```python
from build123d import *

# Parameters (mm, degrees)
F0_R            = 63.5
F0_R_2          = 14.1605
F1_DEPTH        = 3.175
F2_R            = 2.3622
F3_DEPTH        = 3.176
F3_COPIES_COUNT = 6


# Not quite as in the source:
# - a pattern or mirror of a feature is missing from the dataset's text; its kind, count and spacing are read off the source's solid


with BuildPart() as f1:
    # F0 (on Top) → F1 (new body)
    with BuildSketch(Plane.XY):
        Circle(F0_R)
        Circle(F0_R_2, mode=Mode.SUBTRACT)
    extrude(amount=F1_DEPTH)

    # F2 (on face) → F3 (cut, through all)
    with BuildSketch(Plane.XY.offset(3.175)):
        with Locations((0, 23.8125)):
            Circle(F2_R)
        with Locations((25.4, 43.9940905122)):
            Circle(F2_R)
    f3 = extrude(amount=-F3_DEPTH, mode=Mode.SUBTRACT)

    # F3_copies: F3 ×6 about axis
    f3_copies_axis = Axis((0, 0, 0), (0, 0, 1))
    for i in range(1, F3_COPIES_COUNT):
        add(f3.rotate(f3_copies_axis, i * 360 / F3_COPIES_COUNT), mode=Mode.SUBTRACT)


solid = f1.part
```
CAD build for the part. Positions are in the model's coordinates, mm. Round coordinates to 2 decimals unless told otherwise and drop trailing zeros. Loops run counter-clockwise (first coordinate to the right, second up) from the corner with the lowest first, then second, coordinate; pieces in that order, holes last. Notation, with made-up numbers: (82, 63) - (90, 63) arc R22 cw to (90, 75) - close; hole circle Ø2 at (-32.75, 58.25). An arc over 180 degrees is marked (long way). Return JSON: item names as keys, results as strings. Group by question number.
Q1. Band-saw the part on A-A on y = 0. Give the cut face in (x, z) (1 decimal).
Q2. Band-saw the part on B-B on x = 0. Give the cut face in (y, z) (1 decimal).
Q3. Drill centre lines: line 1 along Y through (x, z) = (-25.4, 2.1); line 2 along Y through (x, z) = (20.5, 2); line 3 along X through (y, z) = (43.5, 1.3). Where is each one in solid material? Low to high. Write a range as [from, to].
Q4. Band-saw the part on D-D on y = 38. Give the cut face in (x, z) (3 decimals).
Q5. Two-plate mould, pull along X, no slides. Class faces 1 (the face through (-15, 1, 0)), 2 (the face through (-13.77, -61.99, 1.57)), 3 (the face through (0.308, -26.155, 1.61)): +X half, -X half, draft (parallel to the pull), parting line (faces both ways), or undercut.
Q6. Flat gauge pins, fed straight in: pin 1 Ø4.5 at (x, y) = (-25.4, 43.99) entering from -Z; pin 2 Ø1 at (y, z) = (41, 1) entering from -X; pin 3 Ø1.5 at (x, z) = (-12, 1) entering from +Y. Where does each tip first touch, or does it go through?
Q7. Band-saw the part on C-C on z = 0.85. Give the number of separate pieces and of enclosed holes in the cut face, plus the area to 3 significant figures.
Solutions:
{
 "1": {"outline": "(-63.5, 0) - (-53.2, 0) - (-53.2, 3.2) - (-63.5, 3.2) - close; (-48.4, 0) - (-14.2, 0) - (-14.2, 3.2) - (-48.4, 3.2) - close; (14.2, 0) - (48.4, 0) - (48.4, 3.2) - (14.2, 3.2) - close; (53.2, 0) - (63.5, 0) - (63.5, 3.2) - (53.2, 3.2) - close"},
 "2": {"outline": "(-63.5, 0) - (-26.2, 0) - (-26.2, 3.2) - (-63.5, 3.2) - close; (-21.5, 0) - (-14.2, 0) - (-14.2, 3.2) - (-21.5, 3.2) - close; (14.2, 0) - (21.5, 0) - (21.5, 3.2) - (14.2, 3.2) - close; (26.2, 0) - (63.5, 0) - (63.5, 3.2) - (26.2, 3.2) - close"},
 "3": {"line 1": "y = [-58.2, -46.36], [-41.63, 41.63], [46.36, 58.2]", "line 2": "y = [-60.1, -14.27], [-9.55, 9.55], [14.27, 60.1]", "line 3": "x = [-46.26, -27.71], [-23.09, 23.09], [27.71, 46.26]"},
 "4": {"outline": "(-50.875, 0) - (50.875, 0) - (50.875, 3.175) - (-50.875, 3.175) - close"},
 "5": {"face 1": "draft", "face 2": "parting line", "face 3": "undercut"},
 "6": {"pin 1": "passes through", "pin 2": "stops at x = -48.91", "pin 3": "stops at y = 62.5"},
 "7": {"separate pieces": "1", "enclosed holes": "13", "area": "11,800 mm^2"}
}
